Here's how the part is built. I have some questions about the finished solid (model axes, mm). A direction names the side the tool comes from. Give positions to 0.01 mm unless a question says otherwise; leave off trailing zeros. Write each loop counter-clockwise with the first axis right and the second up, starting at its lowest first coordinate (ties: lowest second). Pieces come first, ordered by that corner, then holes. Notation, with made-up numbers: (77, 20) -> (111, 20) arc R18 cw to (111, 36) -> close; hole circle Ø10 at (37.25, -28). An arc over 180 degrees is marked (long way). Use one line per item in the form item = value.
```python
from build123d import *

# Parameters (mm, degrees)
BOSS_EXTRUDE1_DEPTH     = 50
CUT_EXTRUDE2_DEPTH      = 118.930495595
CUT_EXTRUDE2_DEPTH_BACK = 118.930495595


with BuildPart() as part:
    # Sketch2 → Boss-Extrude1 (new, symmetric)
    with BuildSketch(Plane.XY):
        Polygon((5.01375486, 0), (75.378877849, 0), (75.378877849, -17.541748785), (16.697188205, -17.541748785), (16.697188205, -75.591834267), (0, -75.591834267), (0, -5.01375486), align=None)
    extrude(amount=BOSS_EXTRUDE1_DEPTH, both=True)

    # Sketch6 → Cut-Extrude2 (cut, two sides: drawn at the far end of the back side and taken through both)
    with BuildSketch(Plane(origin=(-2.50687743, -2.50687743, 0), x_dir=(0, 0, 1), z_dir=(0.7071067811865464, 0.7071067811865488, 0)).offset(-CUT_EXTRUDE2_DEPTH_BACK)):
        Polygon((44.940550834, 3.545260061), (50.113588722, 8.718297949), (50.113590784, 3.494380863), align=None)
    extrude(amount=CUT_EXTRUDE2_DEPTH + CUT_EXTRUDE2_DEPTH_BACK, mode=Mode.SUBTRACT)


solid = part.part
```
Q1. Which directions (+Z, -Z, +X, -X, +Y, -Y) give clear straight access to the entire face, cutting with the end or side of a thin tool? Please do faces 1 (the face through (46, -17.542, 1)), 2 (the face through (13, -29, 50)).
Result set:
face_1 = +Z, -Z, +X, -Y
face_2 = +Z, +X, -X, +Y, -Y
Q2. I want a section at B-B, the plane x = 51. Write out the boundary of the cut face in (y, z).
Result set:
outline = (-17.54, -50) -> (0, -50) -> (0, 50) -> (-17.54, 50) -> close
Q3. I want a section at A-A, the plane z = 3.5. Write out the boundary of the cut face in (x, y).
Result set:
outline = (0, -75.59) -> (16.7, -75.59) -> (16.7, -17.54) -> (75.38, -17.54) -> (75.38, 0) -> (5.01, 0) -> (0, -5.01) -> close
Q4. Will this pin go through, and if not, where does the flat tip stop? pin 1 Ø3 at (y, z) = (-65, 11) entering from +X.
Result set:
pin_1 = 16.7
Q5. I want a section at C-C, the plane y = -29.5. Write out the boundary of the cut face in (x, z), and give its area (3 significant figures).
Result set:
outline = (0, -50) -> (16.7, -50) -> (16.7, 50) -> (0, 50) -> close
area = 1,670 mm2
Q6. If I drill on line 1 along X through (y, z) = (-22, -24); line 2 along Y through (x, z) = (52, 31.5); line 3 along Y through (x, z) = (5, 21), over which ranges is the centre line in solid material (lowest first)? Write a range as from..to.
Result set:
line_1 = 0..16.7
line_2 = -17.54..0
line_3 = -75.59..-0.01
